from build123d import *

# Parameters (mm, degrees)
F0_W     = 33
F0_H     = 37
F1_DEPTH = 10
F2_W     = 17.6
F2_H     = 28
F3_DEPTH = 4.2
F4_W     = 1.5
F4_H     = 28
F5_DEPTH = 2.2
F6_R     = 1.25
F7_DEPTH = 10.001


with BuildPart() as f1:
    # F0 (on Top) → F1 (new body)
    with BuildSketch(Plane.XY):
        Rectangle(F0_W, F0_H)
    extrude(amount=F1_DEPTH)

    # F2 (on face) → F3 (cut)
    with BuildSketch(Plane.XY.offset(10)):
        Rectangle(F2_W, F2_H)
        with BuildLine():
            Line((3.2, -6.9), (3.2, -8.25))
            Line((3.2, -8.25), (-3.2, -8.25))
            Line((-3.2, -8.25), (-3.2, -6.9))
            ThreePointArc((-3.2, -6.9), (-1.3, -5), (-3.2, -3.1))
            Line((-3.2, -3.1), (-3.2, -1.9))
            ThreePointArc((-3.2, -1.9), (-1.3, 0), (-3.2, 1.9))
            Line((-3.2, 1.9), (-3.2, 3.1))
            ThreePointArc((-3.2, 3.1), (-1.3, 5), (-3.2, 6.9))
            Line((-3.2, 6.9), (-3.2, 8.25))
            Line((-3.2, 8.25), (3.2, 8.25))
            Line((3.2, 8.25), (3.2, 6.9))
            ThreePointArc((3.2, 6.9), (1.3, 5), (3.2, 3.1))
            Line((3.2, 3.1), (3.2, 1.9))
            ThreePointArc((3.2, 1.9), (1.3, 0), (3.2, -1.9))
            Line((3.2, -1.9), (3.2, -3.1))
            ThreePointArc((3.2, -3.1), (1.3, -5), (3.2, -6.9))
        make_face(mode=Mode.SUBTRACT)
    extrude(amount=-F3_DEPTH, mode=Mode.SUBTRACT)

    # F4 (on face) → F5 (cut)
    with BuildSketch(Plane.XY.offset(10)):
        with Locations((-9.55, 0)):
            Rectangle(F4_W, F4_H)
        with Locations((9.55, 0)):
            Rectangle(F4_W, F4_H)
    extrude(amount=-F5_DEPTH, mode=Mode.SUBTRACT)

    # F6 (on face) → F7 (cut, through all)
    with BuildSketch(Plane.XY.offset(10)):
        with Locations((13.4, 0)):
            Circle(F6_R)
        with Locations((-13.4, 0)):
            Circle(F6_R)
    extrude(amount=-F7_DEPTH, mode=Mode.SUBTRACT)


solid = f1.part
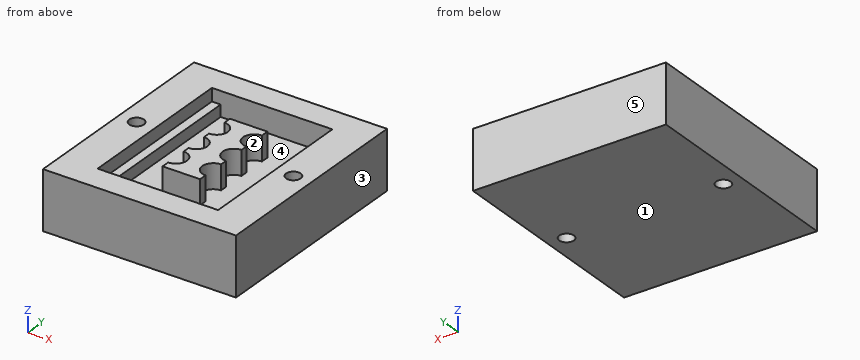
Model file for the job. Use its own axes, mm. Face numbers are marked on the shaded views. A direction names the side the tool comes from. Give positions to 0.01 mm unless a question says otherwise; leave off trailing zeros. Order: outer loops, then holes, each group sorted by start corner. A loop starts at its lowest first (then second) coordinate and runs counter-clockwise, first axis right, second up. Notation, with made-up numbers: M -0.75,10.25 L 26.25,10.25 A22 ccw 26.25,22.25 Z; hole C 30,7.25 d10. An arc over 180 degrees is marked long. Write item = value, one per line.
Q1. Cut at D-D, the plane x = -7.5. List the corners of the cut face in (y, z).
Derived:
outline = M -18.5,0 L 18.5,0 L 18.5,10 L 14,10 L 14,5.8 L -14,5.8 L -14,10 L -18.5,10 Z
Q2. Flat gauge pin, fed straight in: pin 1 (2 mm diameter, centred on x = 12.5, y = 2.5, fed in from -Z). Where does the tip first touch, or does it go through?
Derived:
pin_1 = 0
Q3. Cut at B-B, the plane z = 6.75. List the corners of the cut face in (x, y).
Derived:
outline = M -16.5,-18.5 L 16.5,-18.5 L 16.5,18.5 L -16.5,18.5 Z; M -3.2,-8.25 L 3.2,-8.25 L 3.2,-6.9 A1.9 cw 3.2,-3.1 L 3.2,-1.9 A1.9 cw 3.2,1.9 L 3.2,3.1 A1.9 cw 3.2,6.9 L 3.2,8.25 L -3.2,8.25 L -3.2,6.9 A1.9 cw -3.2,3.1 L -3.2,1.9 A1.9 cw -3.2,-1.9 L -3.2,-3.1 A1.9 cw -3.2,-6.9 Z; hole C -13.4,0 d2.5; hole M -8.8,-14 L 8.8,-14 L 8.8,14 L -8.8,14 Z; hole C 13.4,0 d2.5
Q4. Tool access for the marked faces 1 and 2: list every direction of +Z, -Z, +X, -X, +Y, -Y with a clear straight run to the whole face (end or side of a thin tool).
Derived:
face_1 = -Z, +X, -X, +Y, -Y
face_2 = +Z
Q5. Cut at A-A, the plane x = 13.4. List the corners of the cut face in (y, z).
Derived:
outline = M -18.5,0 L -1.25,0 L -1.25,10 L -18.5,10 Z; M 1.25,0 L 18.5,0 L 18.5,10 L 1.25,10 Z
Q6. Two-plate mould, pull along Y, no slides. Class the marked faces 3, 4 and 5: pulls with the +Y half, pulls with the -Y half, needs draft (parallel to the pull), parting line crosses it, or undercut.
Derived:
face_3 = needs draft
face_4 = undercut
face_5 = pulls with the +Y half
Q7. Cut at C-C, the plane y = 5. List the corners of the cut face in (x, z), then the cut area to 3 significant figures.
Derived:
outline = M -16.5,0 L 16.5,0 L 16.5,10 L 10.3,10 L 10.3,7.8 L 8.8,7.8 L 8.8,5.8 L 1.3,5.8 L 1.3,10 L -1.3,10 L -1.3,5.8 L -8.8,5.8 L -8.8,7.8 L -10.3,7.8 L -10.3,10 L -16.5,10 Z
area = 260 mm2
Q8. Drill centre lines: line 1 (X direction, y = -7.5, z = 6.75); line 2 (X direction, y = 5, z = 8); line 3 (Y direction, x = -6, z = 6.5). Where is each one in solid material? Low to high. Write a range as [from, to].
Derived:
line_1 = [-16.5, -8.8], [-3.2, 3.2], [8.8, 16.5]
line_2 = [-16.5, -10.3], [-1.3, 1.3], [10.3, 16.5]
line_3 = [-18.5, -14], [14, 18.5]
